Build history of the part. All positions in model axes, mm. Face numbers are marked on the shaded views. A direction names the side the tool comes from. Round coordinates to 2 decimals unless told otherwise and drop trailing zeros. Write each loop counter-clockwise with the first axis right and the second up, starting at its lowest first coordinate (ties: lowest second). Pieces come first, ordered by that corner, then holes.
1) Which spindle directions (+Z, -Z, +X, -X, +Y, -Y) get a long thin tool onto all of the face, cutting with end or side? Do the marked faces 3 and 4. Say none if no direction does.
2) Flat gauge pins, fed straight in: pin 1 (8 mm diameter, centred on y = 74.5, z = -14.5, fed in from -X); pin 2 (7.5 mm diameter, centred on x = 63, z = -21.5, fed in from -Y); pin 3 (15 mm diameter, centred on y = 124.5, z = -19, fed in from -X). Where does each tip first touch, or does it go through?
3) Saw through at B-B (y = 163). Write the cut outline in (x, z), plus the area to 3 significant figures.
4) Saw through at D-D (y = 302). Write the cut outline in (x, z).
5) Saw through at A-A (x = 114). Write the cut outline in (y, z).
6) Pull direction Y, two halves, no side cores. Call the marked faces 1 and 2: +Y half, -Y half, draft (parallel to the pull), parting line (faces both ways), or undercut.
7) Wall check: probe 1 along Y at (x, z) = (246, -26); probe 2 along X at (y, z) = (199, -5); probe 3 along Z at (x, y) = (293.5, 195). Give the ranges that are in metal, low to high.
8) Saw through at C-C (x = 259). Write the cut outline in (y, z).
from build123d import *

# Parameters (mm, degrees)
SKETCH1_W           = 398
SKETCH1_H           = 324
BOSS_EXTRUDE1_DEPTH = 23
SKETCH2_W           = 380
SKETCH2_H           = 304
CUT_EXTRUDE1_DEPTH  = 1
SKETCH3_W           = 322
SKETCH3_H           = 162
BOSS_EXTRUDE2_DEPTH = 30
CHAMFER1_SIZE       = 20
CHAMFER1_SIZE2      = 30
SKETCH4_W           = 30
SKETCH4_H           = 10
SKETCH4_W_2         = 35
SKETCH4_H_2         = 26
BOSS_EXTRUDE3_DEPTH = 10
SKETCH5_W           = 15
SKETCH5_H           = 29
CUT_EXTRUDE2_DEPTH  = 25


with BuildPart() as part:
    # Sketch1 → Boss-Extrude1 (new body)
    with BuildSketch(Plane.XY):
        with Locations((199, 162)):
            Rectangle(SKETCH1_W, SKETCH1_H)
    extrude(amount=BOSS_EXTRUDE1_DEPTH)

    # Sketch2 → Cut-Extrude1 (cut)
    with BuildSketch(Plane.XY.offset(23)):
        with Locations((199, 162)):
            Rectangle(SKETCH2_W, SKETCH2_H)
    extrude(amount=-CUT_EXTRUDE1_DEPTH, mode=Mode.SUBTRACT)

    # Sketch3 → Boss-Extrude2 (add)
    with BuildSketch(Plane(origin=(0, 0, 0), x_dir=(-1, 0, 0), z_dir=(0, 0, -1))):
        with Locations((-213, 160)):
            Rectangle(SKETCH3_W, SKETCH3_H)
    extrude(amount=BOSS_EXTRUDE2_DEPTH)

    # Chamfer1
    chamfer1_edges = [part.edges().sort_by_distance(p)[0] for p in [
        (374, 160, -30),
    ]]
    chamfer1_side = [part.faces().sort_by_distance(p)[0] for p in [
        (374, 160, -15),
    ]]
    chamfer(chamfer1_edges, length=CHAMFER1_SIZE, length2=CHAMFER1_SIZE2, reference=chamfer1_side[0])

    # Sketch4 → Boss-Extrude3 (add)
    with BuildSketch(Plane.XZ.offset(-79)):
        with Locations((69, -15)):
            Rectangle(SKETCH4_W, SKETCH4_H)
        with Locations((116.5, -15)):
            Rectangle(SKETCH4_W_2, SKETCH4_H)
        with Locations((304, -15)):
            Rectangle(SKETCH4_W, SKETCH4_H_2)
    extrude(amount=BOSS_EXTRUDE3_DEPTH)

    # Sketch5 → Cut-Extrude2 (cut)
    with BuildSketch(Plane(origin=(0, 0, -30), x_dir=(-1, 0, 0), z_dir=(0, 0, -1))):
        with Locations((-59.5, 120.5)):
            Rectangle(SKETCH5_W, SKETCH5_H)
    extrude(amount=-CUT_EXTRUDE2_DEPTH, mode=Mode.SUBTRACT)


solid = part.part
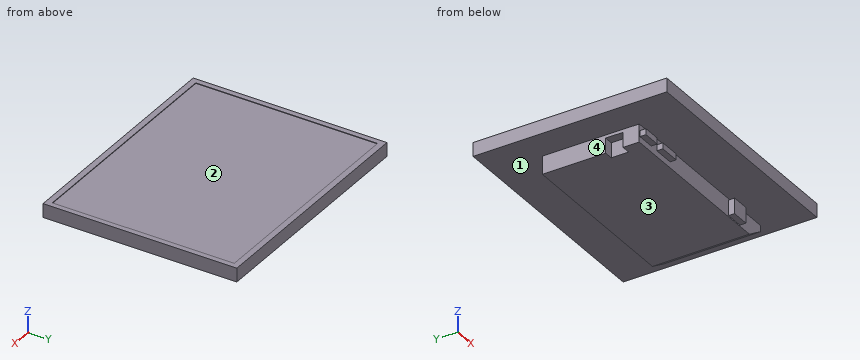
Evaluation:
1. face 3: -Z, +X, -X, +Y, -Y
1. face 4: -Z, -X, +Y, -Y
2. pin 1: stops at x = 54
2. pin 2: stops at y = 69
2. pin 3: stops at x = 67
3. outline: (0, 0) - (52, 0) - (52, -30) - (344, -30) - (374, -10) - (374, 0) - (398, 0) - (398, 23) - (389, 23) - (389, 22) - (9, 22) - (9, 23) - (0, 23) - close
3. area: 18,100 mm2
4. outline: (0, 0) - (398, 0) - (398, 23) - (389, 23) - (389, 22) - (9, 22) - (9, 23) - (0, 23) - close
5. outline: (0, 0) - (79, 0) - (79, -10) - (69, -10) - (69, -20) - (79, -20) - (79, -30) - (241, -30) - (241, 0) - (324, 0) - (324, 23) - (314, 23) - (314, 22) - (10, 22) - (10, 23) - (0, 23) - close
6. face 1: draft
6. face 2: undercut
7. probe 1: y = 79 to 241
7. probe 2: x = 52 to 374
7. probe 3: z = -30 to 22
8. outline: (0, 0) - (79, 0) - (79, -30) - (241, -30) - (241, 0) - (324, 0) - (324, 23) - (314, 23) - (314, 22) - (10, 22) - (10, 23) - (0, 23) - close
